```python
from build123d import *

# Parameters (mm, degrees)
PAD036_DEPTH        = 19.8
POCKET018_DEPTH     = 19.3
SKETCH066_W         = 2
SKETCH066_H         = 4
POCKET019_DEPTH     = 9.9
REVOLUTION001_ANGLE = 12
SKETCH070_R         = 2.95
PAD044_DEPTH        = 1.8
FILLET016_R         = 0.3
FILLET017_R         = 0.8
FILLET018_R         = 0.4


with BuildPart() as part:
    # Sketch050 → Pad036 (new body)
    with BuildSketch(Plane.XZ):
        with BuildLine():
            ThreePointArc((-6.4621977686, 7.5), (-9.9, 0), (-6.4621977686, -7.5))
            Line((-6.4621977686, -7.5), (6.4621977686, -7.5))
            ThreePointArc((6.4621977686, -7.5), (9.9, 0), (6.4621977686, 7.5))
            Line((-6.4621977686, 7.5), (6.4621977686, 7.5))
        make_face()
    extrude(amount=-PAD036_DEPTH)

    # Sketch065 (on Face6 of Pad036) → Pocket018 (cut)
    with BuildSketch(Plane(origin=(0, 19.8, 0), x_dir=(1, 0, 0), z_dir=(0, 1, 0))):
        with BuildLine():
            ThreePointArc((6.3498031466, -7.2), (9.6, 0), (6.3498031466, 7.2))
            Line((-6.3498031466, 7.2), (6.3498031466, 7.2))
            ThreePointArc((-6.3498031466, 7.2), (-9.6, 0), (-6.3498031466, -7.2))
            Line((-6.3498031466, -7.2), (6.3498031466, -7.2))
        make_face()
    extrude(amount=-POCKET018_DEPTH, mode=Mode.SUBTRACT)

    # Sketch066 → Pocket019 (cut, symmetric)
    with BuildSketch(Plane.YZ):
        with Locations((18.8, 0)):
            Rectangle(SKETCH066_W, SKETCH066_H)
    extrude(amount=POCKET019_DEPTH, both=True, mode=Mode.SUBTRACT)

    # Sketch029 → Revolution001 (revolve, symmetric)
    with BuildSketch(Plane.XY) as revolution001_sk:
        with BuildLine():
            Line((-9.2, 18.8), (-8.4, 18.8))
            Line((-8.4, 18.8), (-8.4, 18.5))
            Line((-8.4, 18.5), (-9.2, 18.5))
            ThreePointArc((-9.2, 18.5), (-9.4828427125, 18.3828427125), (-9.6, 18.1))
            Line((-9.6, 18.1), (-9.6, 17.8))
            Line((-9.9, 17.8), (-9.6, 17.8))
            Line((-9.9, 18.1), (-9.9, 17.8))
            ThreePointArc((-9.2, 18.8), (-9.6949747468, 18.5949747468), (-9.9, 18.1))
        make_face()
        with BuildLine():
            Line((9.2, 18.8), (8.4, 18.8))
            Line((8.4, 18.8), (8.4, 18.5))
            Line((8.4, 18.5), (9.2, 18.5))
            ThreePointArc((9.6, 18.1), (9.4828427125, 18.3828427125), (9.2, 18.5))
            Line((9.6, 18.1), (9.6, 17.8))
            Line((9.9, 17.8), (9.6, 17.8))
            Line((9.9, 18.1), (9.9, 17.8))
            ThreePointArc((9.9, 18.1), (9.6949747468, 18.5949747468), (9.2, 18.8))
        make_face()
    revolve(axis=Axis((0, 0, 0), (0, 1, 0)), revolution_arc=REVOLUTION001_ANGLE / 2)
    revolve(revolution001_sk.sketch, axis=Axis((0, 0, 0), (0, -1, 0)), revolution_arc=REVOLUTION001_ANGLE / 2)

    # Sketch070 (on Face5 of Revolution001) → Pad044 (join)
    with BuildSketch(Plane.XZ):
        Circle(SKETCH070_R)
    extrude(amount=PAD044_DEPTH)

    # Fillet016
    fillet016_edges = [part.edges().sort_by_distance(p)[0] for p in [
        (-9.696588, 17.8, -1.019153),
        (-9.542616, 17.8, -2),
        (-9.696588, 17.8, 1.019153),
        (-9.542616, 17.8, 2),
        (-8.353984, 18.65, 0.878039),
        (-8.353984, 18.65, -0.878039),
        (9.542616, 17.8, -2),
        (9.696588, 17.8, -1.019153),
        (9.696588, 17.8, 1.019153),
        (9.542616, 17.8, 2),
        (8.353984, 18.65, 0.878039),
        (8.353984, 18.65, -0.878039),
    ]]
    fillet(fillet016_edges, radius=FILLET016_R)

    # Fillet017
    fillet017_edges = [part.edges().sort_by_distance(p)[0] for p in [
        (9.9, 0, 0),
        (-9.9, 0, 0),
    ]]
    fillet(fillet017_edges, radius=FILLET017_R)

    # Fillet018
    fillet018_edges = [part.edges().sort_by_distance(p)[0] for p in [
        (0, 0, -7.5),
        (0, 0, 7.5),
    ]]
    fillet(fillet018_edges, radius=FILLET018_R)


with BuildPart() as part_1:
    # Body022 placement: moved
    add(part.part.moved(Location((0, 25.7, 0))))


solid = part_1.part
```
Check sheet for the modelled part. Datum: model origin and axes. Units: mm. A direction names the side the tool comes from. Round coordinates to 2 decimals unless told otherwise and drop trailing zeros. Order: outer loops, then holes, each group sorted by start corner. A loop starts at its lowest first (then second) coordinate and runs counter-clockwise, first axis right, second up. Notation, with made-up numbers: M 22,40 L 38,40 A14 ccw 38,65 Z; hole C 46,30.5 d10. An arc over 180 degrees is marked long. Answer in a Markdown table with one row per item.
(1) Section check B-B on y = 40.25. Record the boundary of the cut face in (x, z), plus the area to 3 significant figures.
Findings:
| item | result |
|---|---|
| outline | M -6.58,-7.4 A0.4 ccw -6.31,-7.5 L 6.31,-7.5 A0.4 ccw 6.58,-7.4 A9.9 ccw 6.58,7.4 A0.4 ccw 6.31,7.5 L -6.31,7.5 A0.4 ccw -6.58,7.4 A9.9 ccw Z; hole M -6.35,-7.2 L 6.35,-7.2 A9.6 ccw 6.35,7.2 L -6.35,7.2 A9.6 ccw Z |
| area | 17.7 mm^2 |
(2) Gauge pin test, flat ends, axial feed: pin 1 (1.5 mm diameter, centred on x = 7.5, z = 5.5, fed in from -Y); pin 2 (5 mm diameter, centred on x = 4.5, z = -2, fed in from +Y); pin 3 (1.5 mm diameter, centred on y = 32.5, z = -2, fed in from +X). Record the tip position at first contact, or that the pin passes through.
Findings:
| item | result |
|---|---|
| pin 1 | stops at y = 25.7 |
| pin 2 | stops at y = 26.2 |
| pin 3 | stops at x = 9.82 |
(3) Draft check along Z on faces 6 (the cylindrical face through (9.9, 35.9, -0.1)), 7 (the flat face through (-0.1, 25.7, -3.1)), 8 (the cylindrical face through (9.6, 36, 0.1)). Enter one of: +Z half, -Z half, draft (parallel to the pull), parting line (faces both ways), or undercut.
Findings:
| item | result |
|---|---|
| face 6 | parting line |
| face 7 | draft |
| face 8 | undercut |
(4) Set-up check for faces 1 (the flat face through (0, 36, 7.2)), 2 (the flat face through (-9, 44.2, 0)), 3 (the flat face through (-9, 44.5, 0)), 4 (the flat face through (0, 36, 7.5)), 5 (the cylindrical face through (-2.947, 24.813, 0.13)): record each of +Z, -Z, +X, -X, +Y, -Y from which the full face is reachable in a straight line by a thin tool's end or side.
Findings:
| item | result |
|---|---|
| face 1 | +Y |
| face 2 | none |
| face 3 | +X, -X, +Y |
| face 4 | +Z, +X, -X, +Y, -Y |
| face 5 | -Y |
(5) Section check A-A on z = 0. Record the boundary of the cut face in (x, y).
Findings:
| item | result |
|---|---|
| outline | M -9.9,26.5 A0.8 ccw -9.1,25.7 L -2.95,25.7 L -2.95,23.9 L 2.95,23.9 L 2.95,25.7 L 9.1,25.7 A0.8 ccw 9.9,26.5 L 9.9,43.8 A0.7 ccw 9.2,44.5 L 8.4,44.5 L 8.4,44.2 L 9.2,44.2 A0.4 cw 9.6,43.8 L 9.6,26.2 L -9.6,26.2 L -9.6,43.8 A0.4 cw -9.2,44.2 L -8.4,44.2 L -8.4,44.5 L -9.2,44.5 A0.7 ccw -9.9,43.8 Z |
(6) Section check C-C on x = 0. Record the boundary of the cut face in (y, z), plus the area to 3 significant figures.
Findings:
| item | result |
|---|---|
| outline | M 23.9,-2.95 L 25.7,-2.95 L 25.7,-7.1 A0.4 ccw 26.1,-7.5 L 45.5,-7.5 L 45.5,-7.2 L 26.2,-7.2 L 26.2,7.2 L 45.5,7.2 L 45.5,7.5 L 26.1,7.5 A0.4 ccw 25.7,7.1 L 25.7,2.95 L 23.9,2.95 Z |
| area | 29.6 mm^2 |
(7) Material ranges on line 1 along Z through (x, y) = (6, 26.75); line 2 along X through (y, z) = (35, 0.25); line 3 along X through (y, z) = (27, -2), recorded low to high. Write a range as from..to.
Findings:
| item | result |
|---|---|
| line 1 | z = -7.5..-7.2, 7.2..7.5 |
| line 2 | x = -9.9..-9.6, 9.6..9.9 |
| line 3 | x = -9.7..-9.39, 9.39..9.7 |
